Could you check a few things on this model? Use its own coordinates, in mm. Face numbers are marked on the shaded views. A direction names the side the tool comes from. Round coordinates to 2 decimals unless told otherwise and drop trailing zeros. Loops run counter-clockwise (first coordinate to the right, second up) from the corner with the lowest first, then second, coordinate; pieces in that order, holes last. Notation, with made-up numbers: M 76,30 L 81,30 A19 ccw 81,67 Z; hole C 81.25,56 d8. An arc over 180 degrees is marked long. One line per item, written item: value. Start each with the question number.
Q1. Imagine slicing it at B-B (x = -13.5). Please give me the cut outline in (y, z), then the cut area to 3 significant figures.
Q2. Which directions (+Z, -Z, +X, -X, +Y, -Y) give clear straight access to the entire face, cutting with the end or side of a thin tool? Please do the marked faces 1 and 2.
Q3. I'm going to push flat-ended pins straight in: pin 1 Ø1.5 at (y, z) = (181.5, -12.5) entering from +X; pin 2 Ø6 at (x, z) = (44, -15.5) entering from +Y; pin 3 Ø5 at (x, y) = (-11, 141.5) entering from -Z. Where does each tip first touch, or does it pass through?
Q4. Imagine slicing it at C-C (y = 37). Please give me the cut outline in (x, z) (3 decimals), then the cut area to 3 significant figures.
Q5. Imagine slicing it at A-A (y = 161). Please give me the cut outline in (x, z) (3 decimals), then the cut area to 3 significant figures.
Q6. Please list where these lines run through material, in increasing order: line 1 along Z through (x, y) = (-53, 217); line 2 along X through (y, z) = (16.5, -16.75); line 3 along Z through (x, y) = (44.5, 160).
from build123d import *

# Parameters (mm, degrees)
BOSS_EXTRUDE1_DEPTH = 228.6
SKETCH2_W           = 25.4
SKETCH2_H           = 25.4
SKETCH2_H_2         = 19.05
BOSS_EXTRUDE2_DEPTH = 6.35
SKETCH3_W           = 25.4
SKETCH3_H           = 25.4
CUT_EXTRUDE1_DEPTH  = 228.6
SKETCH4_W           = 16.326805286
SKETCH4_H           = 25.4
BOSS_EXTRUDE3_DEPTH = 6.35


with BuildPart() as part:
    # Sketch1 → Boss-Extrude1 (new body)
    with BuildSketch(Plane(origin=(0, 0, 0), x_dir=(1, 0, 0), z_dir=(0, 1, 0))):
        Polygon((-53.975, 0), (53.975, 0), (34.517471145, 16.326805286), (-53.975, 16.326805286), align=None)
    extrude(amount=BOSS_EXTRUDE1_DEPTH)

    # Sketch2 → Boss-Extrude2 (add)
    with BuildSketch(Plane(origin=(22.301169805, 0, -26.577499234), x_dir=(-0.7660444431189819, 0, -0.6427876096865348), z_dir=(0.6427876096865348, 0, -0.7660444431189819))):
        with Locations((-28.647248817, 209.55)):
            Rectangle(SKETCH2_W, SKETCH2_H)
        with Locations((-28.647248817, 158.75)):
            Rectangle(SKETCH2_W, SKETCH2_H)
        with Locations((-28.647248817, 107.95)):
            Rectangle(SKETCH2_W, SKETCH2_H)
        with Locations((-28.647248817, 57.15)):
            Rectangle(SKETCH2_W, SKETCH2_H)
        with Locations((-28.647248817, 9.525)):
            Rectangle(SKETCH2_W, SKETCH2_H_2)
    extrude(amount=BOSS_EXTRUDE2_DEPTH)

    # Sketch3 → Cut-Extrude1 (cut)
    with BuildSketch(Plane(origin=(0, 228.6, 0), x_dir=(1, 0, 0), z_dir=(0, 1, 0))):
        with Locations((66.675, 12.7)):
            Rectangle(SKETCH3_W, SKETCH3_H)
    extrude(amount=-CUT_EXTRUDE1_DEPTH, mode=Mode.SUBTRACT)

    # Sketch4 → Boss-Extrude3 (add)
    with BuildSketch(Plane.ZY.offset(53.975)):
        with Locations((-8.163402643, 12.7)):
            Rectangle(SKETCH4_W, SKETCH4_H)
        with Locations((-8.163402643, 63.5)):
            Rectangle(SKETCH4_W, SKETCH4_H)
        with Locations((-8.163402643, 114.3)):
            Rectangle(SKETCH4_W, SKETCH4_H)
        with Locations((-8.163402643, 165.1)):
            Rectangle(SKETCH4_W, SKETCH4_H)
        with Locations((-8.163402643, 215.9)):
            Rectangle(SKETCH4_W, SKETCH4_H)
    extrude(amount=BOSS_EXTRUDE3_DEPTH)


solid = part.part
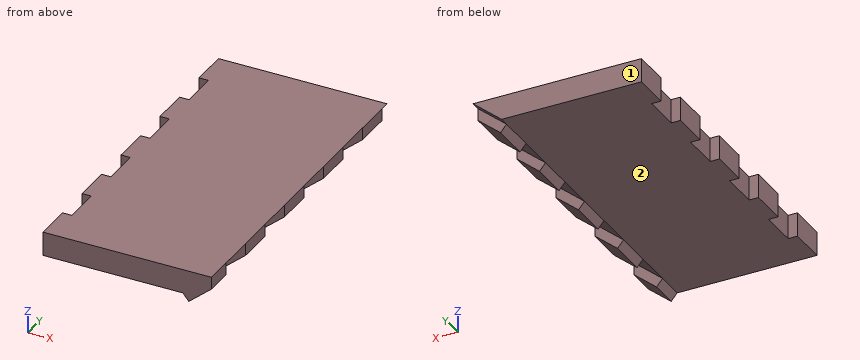
Report:
1. outline: M 0,-16.33 L 228.6,-16.33 L 228.6,0 L 0,0 Z
1. area: 3,730 mm²
2. face 1: +Z, -Z, +X, -X, +Y
2. face 2: -Z, -X, +Y, -Y
3. pin 1: stops at x = 39.97
3. pin 2: stops at y = 222.25
3. pin 3: stops at z = -16.33
4. outline: M -53.975,-16.327 L 34.517,-16.327 L 53.975,0 L -53.975,0 Z
4. area: 1,600 mm²
5. outline: M -60.325,-16.327 L 34.517,-16.327 L 38.599,-21.191 L 53.975,-8.289 L 53.975,0 L -60.325,0 Z
5. area: 1,850 mm²
6. line 1: z = -16.33 to 0
6. line 2: x = 34.87 to 43.89
6. line 3: z = -16.24 to 0
